Input: part model. Units: mm. Frame: model coordinates. A direction names the side the tool comes from. Coordinates: 2 decimals unless noted, no trailing zeros. Order: outer loops, then holes, each group sorted by start corner. A loop starts at its lowest first (then second) coordinate and runs counter-clockwise, first axis right, second up. Notation, with made-up numbers: (36.25, -2) -> (48.25, -2) arc R23 ccw to (48.25, 9) -> close; hole circle Ø2 at (-13.5, 15.25). An arc over 180 degrees is marked (long way). Use one line per item in the form item = value. Start each with the question number.
1) Ray query, line 1 along Y through (x, z) = (18, 0.5); line 2 along Y through (x, z) = (4.25, 11.25); line 3 along Z through (x, y) = (10.5, 0.5). Return the intervals inside material, ascending.
2) Section query C-C on z = 10. Count the separate pieces of the cut face and the enclosed holes in it, then the cut area to 3 significant figures.
3) Access query for faces 1 (the flat face through (13, 0.99, 8.07)), 2 (the flat face through (12, 0, 2)), 3 (the flat face through (18.9, -1.6, 2.5)), 4 (the flat face through (15, -3, 1)), 5 (the flat face through (18, 8, 14)). Directions: +Z, -Z, +X, -X, +Y, -Y. A direction counts if a zero-diameter tool reaches every point of the face in a straight line with its end or side. Return the directions, or none.
4) Section query A-A on y = 13.5. Output: boundary loops of the cut face in (x, z).
5) Pin query (flat end, axial travel): pin 1 (2 mm diameter, centred on x = 24.5, z = 2, fed in from +Y); pin 2 (2 mm diameter, centred on y = 11, z = 14, fed in from +X); pin 3 (1.2 mm diameter, centred on x = 18, y = 18, fed in from +Z); pin 4 (0.6 mm diameter, centred on y = 15, z = 7.5, fed in from -X). Return the tip coordinate at first contact, or that it passes through.
6) Draft query along X for faces 6 (the flat face through (21, 19, 1)), 7 (the cylindrical face through (1, 7.9, 11.5)), 8 (the cylindrical face through (0.57, 0.6, 6.59)), 9 (the flat face through (10, 19, 1)). Return one class per face: pulls with the +X half, pulls with the -X half, needs draft (parallel to the pull), parting line crosses it, or undercut.
7) Section query B-B on y = -3. Output: boundary loops of the cut face in (x, z), then the cut area to 3 significant figures.
from build123d import *

# Parameters (mm, degrees)
CROQUIS1_W              = 23
CROQUIS1_H              = 16
SALIENTE_EXTRUIR1_DEPTH = 15
CROQUIS2_W              = 11
CROQUIS2_H              = 12
CORTAR_EXTRUIR1_DEPTH   = 21
CORTAR_EXTRUIR2_DEPTH   = 23
CROQUIS5_W              = 5
CROQUIS5_H              = 12
CORTAR_EXTRUIR3_DEPTH   = 2
REDONDEO1_R             = 2
CORTAR_EXTRUIR4_DEPTH   = 32.780497164
CROQUIS18_W             = 21
CROQUIS18_H             = 12
CORTAR_EXTRUIR8_DEPTH   = 31.886890423
CROQUIS17_W             = 15
CROQUIS17_H             = 16
SALIENTE_EXTRUIR7_DEPTH = 2
REDONDEO8_R             = 2
CROQUIS19_W             = 6
CROQUIS19_H             = 2.5
SALIENTE_EXTRUIR8_DEPTH = 6
CROQUIS20_W             = 6
CROQUIS20_H             = 2.5
SALIENTE_EXTRUIR9_DEPTH = 6
CROQUIS21_R             = 1.5
CORTAR_EXTRUIR9_DEPTH   = 36.570352824
REDONDEO9_R             = 1
CORTAR_EXTRUIR10_DEPTH  = 16
CORTAR_EXTRUIR11_DEPTH  = 2


with BuildPart() as part:
    # Croquis1 → Saliente-Extruir1 (new body)
    with BuildSketch(Plane.XY):
        with Locations((11.5, 8)):
            Rectangle(CROQUIS1_W, CROQUIS1_H)
    extrude(amount=SALIENTE_EXTRUIR1_DEPTH)

    # Croquis2 → Cortar-Extruir1 (cut)
    with BuildSketch(Plane(origin=(23, 0, 0), x_dir=(0, 0, -1), z_dir=(1, 0, 0))):
        with Locations((-7.5, 8)):
            Rectangle(CROQUIS2_W, CROQUIS2_H)
    extrude(amount=-CORTAR_EXTRUIR1_DEPTH, mode=Mode.SUBTRACT)

    # Croquis4 → Cortar-Extruir2 (cut)
    with BuildSketch(Plane.ZY):
        with BuildLine():
            Line((7.5, 12), (0, 12))
            Line((0, 12), (0, 4))
            Line((0, 4), (7.5, 4))
            ThreePointArc((7.5, 4), (11.5, 8), (7.5, 12))
        make_face()
    extrude(amount=-CORTAR_EXTRUIR2_DEPTH, mode=Mode.SUBTRACT)

    # Croquis5 → Cortar-Extruir3 (cut)
    with BuildSketch(Plane.XY.offset(15)):
        with Locations((20.5, 8)):
            Rectangle(CROQUIS5_W, CROQUIS5_H)
    extrude(amount=-CORTAR_EXTRUIR3_DEPTH, mode=Mode.SUBTRACT)

    # Redondeo1
    redondeo1_edges = [part.edges().sort_by_distance(p)[0] for p in [
        (11.5, 16, 15),
        (11.5, 0, 15),
        (0, 16, 7.5),
        (0, 8, 15),
        (0, 0, 7.5),
    ]]
    fillet(redondeo1_edges, radius=REDONDEO1_R)

    # Croquis8 → Cortar-Extruir4 (cut, through all)
    with BuildSketch(Plane.XY.offset(15)):
        Polygon((16.5, 3), (16.5, 13), (3, 8), align=None)
        Polygon((3, 6.500458737), (3, 3), (13, 3), align=None)
        Polygon((3, 9.5), (3, 13), (13, 13), align=None)
    extrude(amount=-CORTAR_EXTRUIR4_DEPTH, mode=Mode.SUBTRACT)

    # Croquis18 → Cortar-Extruir8 (cut, through all)
    with BuildSketch(Plane.XY.offset(2)):
        with Locations((12.5, 8)):
            Rectangle(CROQUIS18_W, CROQUIS18_H)
    extrude(amount=-CORTAR_EXTRUIR8_DEPTH, mode=Mode.SUBTRACT)

    # Croquis17 → Saliente-Extruir7 (add)
    with BuildSketch(Plane(origin=(23, 0, 0), x_dir=(0, 0, -1), z_dir=(1, 0, 0))):
        with Locations((-7.5, 8)):
            Rectangle(CROQUIS17_W, CROQUIS17_H)
    extrude(amount=SALIENTE_EXTRUIR7_DEPTH)

    # Redondeo8
    # the kernel refuses this fillet: 2 mm, written as the material it takes off along each edge
    with BuildSketch(Plane(origin=(23, 14, 13), x_dir=(1, 0, 0), z_dir=(0, 1, 0))) as redondeo8_piece_1_section:
        Polygon((0, 0), (REDONDEO8_R * 1.02, 0), (REDONDEO8_R * 1.02, -REDONDEO8_R * 1.02), (0, -REDONDEO8_R * 1.02), align=None)
    redondeo8_piece_1 = extrude(amount=REDONDEO8_R * 1.02, mode=Mode.PRIVATE)
    redondeo8_piece_1 = redondeo8_piece_1 - Plane(origin=(23, 14, 13), x_dir=(-0.7071067811865475, 0, -0.7071067811865475), z_dir=(0, 1, 0)) * Sphere(REDONDEO8_R, mode=Mode.PRIVATE)
    add(redondeo8_piece_1, mode=Mode.SUBTRACT)
    with BuildSketch(Plane(origin=(23, 2, 13), x_dir=(1, 0, 0), z_dir=(0, -1, 0))) as redondeo8_piece_2_section:
        Polygon((0, 0), (REDONDEO8_R * 1.02, 0), (REDONDEO8_R * 1.02, REDONDEO8_R * 1.02), (0, REDONDEO8_R * 1.02), align=None)
    redondeo8_piece_2 = extrude(amount=REDONDEO8_R * 1.02, mode=Mode.PRIVATE)
    redondeo8_piece_2 = redondeo8_piece_2 - Plane(origin=(23, 2, 13), x_dir=(-0.7071067811865475, 0, -0.7071067811865475), z_dir=(0, -1, 0)) * Sphere(REDONDEO8_R, mode=Mode.PRIVATE)
    add(redondeo8_piece_2, mode=Mode.SUBTRACT)
    with BuildSketch(Plane(origin=(23, 14, 15), x_dir=(0, 0, -1), z_dir=(0, 1, 0))) as redondeo8_piece_3_section:
        with BuildLine():
            CenterArc((REDONDEO8_R, -REDONDEO8_R), REDONDEO8_R, 90, 90)
            Line((0, -REDONDEO8_R), (0, 0))
            Line((0, 0), (REDONDEO8_R, 0))
        make_face()
    redondeo8_piece_3 = extrude(amount=7, mode=Mode.PRIVATE)
    redondeo8_piece_3 = redondeo8_piece_3 - Plane(origin=(23.57115566, 14, 13), x_dir=(0, 0, 1), z_dir=(-1, 0, 0)) * Cylinder(2, 23, mode=Mode.PRIVATE)
    add(redondeo8_piece_3, mode=Mode.SUBTRACT)
    with BuildSketch(Plane(origin=(23, -5, 15), x_dir=(1, 0, 0), z_dir=(0, 1, 0))) as redondeo8_piece_4_section:
        with BuildLine():
            CenterArc((REDONDEO8_R, REDONDEO8_R), REDONDEO8_R, 180, 90)
            Line((0, REDONDEO8_R), (0, 0))
            Line((0, 0), (REDONDEO8_R, 0))
        make_face()
    redondeo8_piece_4 = extrude(amount=7, mode=Mode.PRIVATE)
    redondeo8_piece_4 = redondeo8_piece_4 - Plane(origin=(23.571155663, 2, 13), x_dir=(0, -1, 0), z_dir=(1, 0, 0)) * Cylinder(2, 22, mode=Mode.PRIVATE)
    add(redondeo8_piece_4, mode=Mode.SUBTRACT)
    with BuildSketch(Plane(origin=(25, 16, 13), x_dir=(-1, 0, 0), z_dir=(0, 0, -1)), Plane(origin=(25, 0, -5), x_dir=(-1, 0, 0), z_dir=(0, 0, 1))) as redondeo8_piece_5:
        with BuildLine():
            CenterArc((REDONDEO8_R, -REDONDEO8_R), REDONDEO8_R, 90, 90)
            Line((0, -REDONDEO8_R), (0, 0))
            Line((0, 0), (REDONDEO8_R, 0))
        make_face()
    extrude(amount=18, mode=Mode.SUBTRACT)
    with BuildSketch(Plane(origin=(25, 2, 15), x_dir=(0, 0, -1), z_dir=(0, 1, 0))) as redondeo8_piece_6:
        with BuildLine():
            CenterArc((REDONDEO8_R, REDONDEO8_R), REDONDEO8_R, 180, 90)
            Line((0, REDONDEO8_R), (0, 0))
            Line((0, 0), (REDONDEO8_R, 0))
        make_face()
    extrude(amount=12, mode=Mode.SUBTRACT)

    # Croquis19 → Saliente-Extruir8 (add)
    with BuildSketch(Plane(origin=(0, 16, 0), x_dir=(1, 0, 0), z_dir=(0, 1, 0))):
        with Locations((18, -1.25)):
            Rectangle(CROQUIS19_W, CROQUIS19_H)
        with Locations((7, -1.25)):
            Rectangle(CROQUIS19_W, CROQUIS19_H)
    extrude(amount=SALIENTE_EXTRUIR8_DEPTH)

    # Croquis20 → Saliente-Extruir9 (add)
    with BuildSketch(Plane.XZ):
        with Locations((7, 1.25)):
            Rectangle(CROQUIS20_W, CROQUIS20_H)
        with Locations((18, 1.25)):
            Rectangle(CROQUIS20_W, CROQUIS20_H)
    extrude(amount=SALIENTE_EXTRUIR9_DEPTH)

    # Croquis21 → Cortar-Extruir9 (cut, through all)
    with BuildSketch(Plane.XY.offset(2.5)):
        with Locations((18, 19)):
            Circle(CROQUIS21_R)
        with Locations((7, 19)):
            Circle(CROQUIS21_R)
        with Locations((7, -3)):
            Circle(CROQUIS21_R)
        with Locations((18, -3)):
            Circle(CROQUIS21_R)
    extrude(amount=-CORTAR_EXTRUIR9_DEPTH, mode=Mode.SUBTRACT)

    # Redondeo9
    redondeo9_edges = [part.edges().sort_by_distance(p)[0] for p in [
        (21, 16, 1.25),
        (21, 19, 2.5),
        (15, 16, 1.25),
        (18, 16, 2.5),
        (15, 19, 2.5),
        (21, 22, 1.25),
        (15, 22, 1.25),
        (18, 22, 2.5),
        (4, 16, 1.25),
        (7, 16, 2.5),
        (4, 19, 2.5),
        (10, 16, 1.25),
        (10, 19, 2.5),
        (4, 22, 1.25),
        (7, 22, 2.5),
        (10, 22, 1.25),
        (4, 0, 1.25),
        (4, -3, 2.5),
        (10, 0, 1.25),
        (7, 0, 2.5),
        (10, -3, 2.5),
        (4, -6, 1.25),
        (10, -6, 1.25),
        (7, -6, 2.5),
        (21, 0, 1.25),
        (18, 0, 2.5),
        (21, -3, 2.5),
        (15, 0, 1.25),
        (15, -3, 2.5),
        (21, -6, 1.25),
        (18, -6, 2.5),
        (15, -6, 1.25),
    ]]
    fillet(redondeo9_edges, radius=REDONDEO9_R)

    # Croquis22 → Cortar-Extruir10 (cut)
    with BuildSketch(Plane.XZ):
        Polygon((3, 11.25), (21.25, 3.5), (3, 3.5), align=None)
        Polygon((22, 4.25), (3.75, 12), (22, 12), align=None)
    extrude(amount=-CORTAR_EXTRUIR10_DEPTH, mode=Mode.SUBTRACT)

    # Croquis23 → Cortar-Extruir11 (cut)
    with BuildSketch(Plane(origin=(25, 0, 0), x_dir=(0, 0, -1), z_dir=(1, 0, 0))):
        with BuildLine():
            Line((0, 4), (0, 12))
            Line((0, 12), (-6.5, 12))
            ThreePointArc((-6.5, 12), (-10.5, 8), (-6.5, 4))
            Line((-6.5, 4), (0, 4))
        make_face()
    extrude(amount=-CORTAR_EXTRUIR11_DEPTH, mode=Mode.SUBTRACT)


solid = part.part
Answers below:
q1.line_1 = -6 to -4.5, -1.5 to 2, 14 to 17.5, 20.5 to 22
q1.line_2 = 0 to 2, 14 to 16
q1.line_3 = 0 to 3.5, 8.07 to 9.13, 12 to 14.32
q2.separate_pieces = 6
q2.enclosed_holes = 0
q2.area = 58.4 mm^2
q3.face_1 = +Y, -Y
q3.face_2 = +Z, -Y
q3.face_3 = +Z, +X, -X, -Y
q3.face_4 = +Z, -Z, -Y
q3.face_5 = +Z, -Z
q4.outline = (0, 0) -> (2, 0) -> (2, 13) -> (18, 13) -> (18, 15) -> (2, 15) arc R2 ccw to (0, 13) -> close; (23, 0) -> (25, 0) -> (25, 13) arc R2 ccw to (23, 15) -> close
q5.pin_1 = 15.94
q5.pin_2 = 25
q5.pin_3 = 2.5
q5.pin_4 = 0.13
q6.face_6 = pulls with the +X half
q6.face_7 = needs draft
q6.face_8 = pulls with the -X half
q6.face_9 = undercut
q7.outline = (4, 0) -> (5.5, 0) -> (5.5, 2.5) -> (5, 2.5) arc R1 ccw to (4, 1.5) -> close; (8.5, 0) -> (10, 0) -> (10, 1.5) arc R1 ccw to (9, 2.5) -> (8.5, 2.5) -> close; (15, 0) -> (16.5, 0) -> (16.5, 2.5) -> (16, 2.5) arc R1 ccw to (15, 1.5) -> close; (19.5, 0) -> (21, 0) -> (21, 1.5) arc R1 ccw to (20, 2.5) -> (19.5, 2.5) -> close
q7.area = 14.1 mm^2
